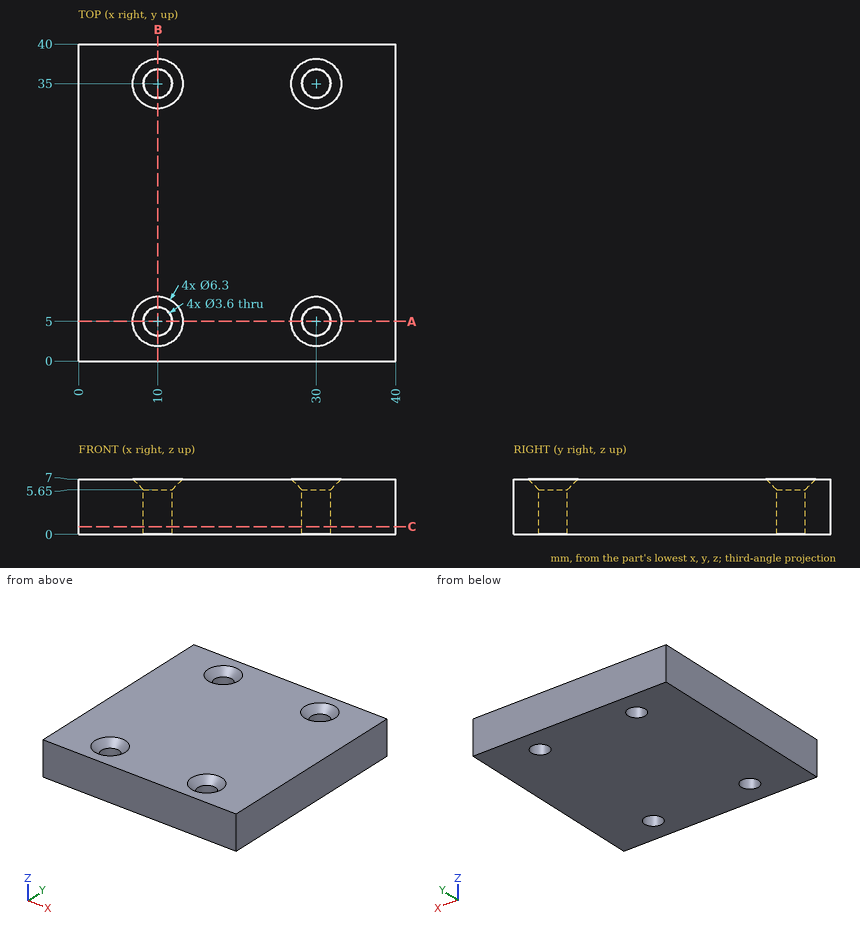
Check sheet for the drawn part. Datum: minimum x, y, z corner. Units: mm. Round coordinates to 2 decimals unless told otherwise and drop trailing zeros. Order: outer loops, then holes, each group sorted by start corner. A loop starts at its lowest first (then second) coordinate and runs counter-clockwise, first axis right, second up.
1) Section check A-A (y = 5). Record the boundary of the cut face in (x, z).
2) Go/stop test with flat-tipped pins: pin 1 Ø4 at (x, y) = (10, 5) entering from +Z; pin 2 Ø3 at (x, y) = (10, 35) entering from -Z. Record where each tip stops, or that it passes through.
3) Scan lines: line 1 (Y direction, x = 30, z = 1.3); line 2 (X direction, y = 35, z = 3.1); line 3 (Y direction, x = 11.5, z = 6). Record each from-to range of solid material in increasing order.
4) Section check C-C (z = 1). Record the boundary of the cut face in (x, y).
5) Section check B-B (x = 10). Record the boundary of the cut face in (y, z), and give its area (3 significant figures).
Result:
1. outline: (0, 0) - (8.2, 0) - (8.2, 5.65) - (6.85, 7) - (0, 7) - close; (11.8, 0) - (28.2, 0) - (28.2, 5.65) - (26.85, 7) - (13.15, 7) - (11.8, 5.65) - close; (31.8, 0) - (40, 0) - (40, 7) - (33.15, 7) - (31.8, 5.65) - close
2. pin 1: stops at z = 5.85
2. pin 2: passes through
3. line 1: y = 0 to 3.2, 6.8 to 33.2, 36.8 to 40
3. line 2: x = 0 to 8.2, 11.8 to 28.2, 31.8 to 40
3. line 3: y = 0 to 3.46, 6.54 to 33.46, 36.54 to 40
4. outline: (0, 0) - (40, 0) - (40, 40) - (0, 40) - close; hole circle Ø3.6 at (10, 5); hole circle Ø3.6 at (10, 35); hole circle Ø3.6 at (30, 5); hole circle Ø3.6 at (30, 35)
5. outline: (0, 0) - (3.2, 0) - (3.2, 5.65) - (1.85, 7) - (0, 7) - close; (6.8, 0) - (33.2, 0) - (33.2, 5.65) - (31.85, 7) - (8.15, 7) - (6.8, 5.65) - close; (36.8, 0) - (40, 0) - (40, 7) - (38.15, 7) - (36.8, 5.65) - close
5. area: 226 mm2
